Geometry: final body of the model. Coordinates: model frame, mm. Round coordinates to 2 decimals unless told otherwise and drop trailing zeros. Loops run counter-clockwise (first coordinate to the right, second up) from the corner with the lowest first, then second, coordinate; pieces in that order, holes last. Notation, with made-up numbers: (15, -40) - (63, -40) arc R22 ccw to (63, -8) - close; hole circle Ø7 at (49, 83.5). An arc over 180 degrees is marked (long way). Answer as a JSON object with one key per item and string values. Group by question number.
Item 1: First-contact query: pin 1 (1 mm diameter, centred on x = 4, y = 4.5, fed in from -Z). Flat tip, straight axial feed; report the tip coordinate or a pass-through.
Item 2: Line query: line 1 (Y direction, x = 0, z = 1.05); line 2 (X direction, y = -3.5, z = 0.5); line 3 (X direction, y = -6.5, z = 1.5). Output: solid intervals per line, ascending.
Item 3: Section D-D (z = 0.4). Return the cut outline in (x, y).
Item 4: Section C-C (z = 1.55). Return the cut outline in (x, y), plus the area to 3 significant figures.
```python
from build123d import *

# Parameters (mm, degrees)
SKETCH1_R           = 9
BOSS_EXTRUDE1_DEPTH = 2
SKETCH2_R           = 7
CUT_EXTRUDE1_DEPTH  = 2
FILLET1_R           = 1


with BuildPart() as part:
    # Sketch1 → Boss-Extrude1 (new body)
    with BuildSketch(Plane.XY):
        Circle(SKETCH1_R)
    extrude(amount=BOSS_EXTRUDE1_DEPTH)

    # Sketch2 → Cut-Extrude1 (cut)
    with BuildSketch(Plane.XY.offset(2)):
        Circle(SKETCH2_R)
    extrude(amount=-CUT_EXTRUDE1_DEPTH, mode=Mode.SUBTRACT)

    # Fillet1
    fillet1_edges = [part.edges().sort_by_distance(p)[0] for p in [
        (-9, 0, 0),
        (-9, 0, 2),
        (-7, 0, 0),
        (-7, 0, 2),
    ]]
    fillet(fillet1_edges, radius=FILLET1_R - 0.0001)  # a hair under: the kernel refuses the full size


solid = part.part
```
Values:
{
 "1": {"pin 1": "passes through"},
 "2": {"line 1": "y = -9 to -7, 7 to 9", "line 2": "x = -8.15 to -6.22, 6.22 to 8.15", "line 3": "x = -6.03 to -2.94, 2.94 to 6.03"},
 "3": {"outline": "circle Ø17.6 at (0, 0); hole circle Ø14.4 at (0, 0)"},
 "4": {"outline": "circle Ø17.67 at (0, 0); hole circle Ø14.33 at (0, 0)", "area": "84.0 mm^2"}
}
